from build123d import *

# Parameters (mm, degrees)
BOSS_EXTRUDE1_DEPTH = 16
SKETCH2_W           = 9
SKETCH2_H           = 16
BOSS_EXTRUDE2_DEPTH = 1
BOSS_EXTRUDE2_TAPER = 45
SKETCH3_R           = 2.6
CUT_EXTRUDE1_DEPTH  = 6
SKETCH4_R           = 1.44
BOSS_EXTRUDE3_DEPTH = 6


with BuildPart() as part:
    # Sketch1 → Boss-Extrude1 (new body)
    with BuildSketch(Plane(origin=(0, 0, 0), x_dir=(1, 0, 0), z_dir=(0, 1, 0))):
        Polygon((-6.542273602, -4.737945966), (13.457726398, -4.737945966), (9.36611498, -0.737945966), (-2.80088502, -0.737945966), align=None)
    extrude(amount=-BOSS_EXTRUDE1_DEPTH)

    # Sketch2 → Boss-Extrude2 (add)
    with BuildSketch(Plane.XY.offset(4.737945966)):
        with Locations((3.457726398, -8)):
            Rectangle(SKETCH2_W, SKETCH2_H)
    extrude(amount=BOSS_EXTRUDE2_DEPTH, taper=BOSS_EXTRUDE2_TAPER)

    # Sketch3 → Cut-Extrude1 (cut, through all)
    with BuildSketch(Plane.XY.offset(5.737945966)):
        with Locations((3.457726398, -5)):
            Circle(SKETCH3_R)
    extrude(amount=-CUT_EXTRUDE1_DEPTH, mode=Mode.SUBTRACT)

    # Sketch4 → Boss-Extrude3 (add)
    with BuildSketch(Plane.XZ.offset(16)):
        with BuildLine():
            Line((13.457726398, 4.737945966), (13.457726398, -6.650054034))
            ThreePointArc((13.457726398, -6.650054034), (10.961456039, -10.319414663), (6.631765726, -9.345066204))
            Line((6.631765726, -9.345066204), (-6.542273602, 4.737945966))
            Line((-6.542273602, 4.737945966), (13.457726398, 4.737945966))
        make_face()
        with Locations((9.512726398, -6.650054034)):
            Circle(SKETCH4_R, mode=Mode.SUBTRACT)
    extrude(amount=-BOSS_EXTRUDE3_DEPTH)


solid = part.part
CAD build for the part. Positions are in the model's coordinates, mm. A direction names the side the tool comes from. Give positions to 0.01 mm unless a question says otherwise; leave off trailing zeros. Write each loop counter-clockwise with the first axis right and the second up, starting at its lowest first coordinate (ties: lowest second). Pieces come first, ordered by that corner, then holes. Notation, with made-up numbers: (77, -24) -> (125, -24) arc R32 ccw to (125, 11) -> close; hole circle Ø6 at (-19, -8.75). An arc over 180 degrees is marked (long way). Return JSON: item names as keys, results as strings.
Item 1: Band-saw the part on A-A (y = -5). List the corners of the cut face in (x, z), then the cut area to 3 significant figures.
Answer below:
{"outline": "(-6.54, 4.74) -> (-2.8, 0.74) -> (0.86, 0.74) -> (0.86, 5.74) -> (-0.04, 5.74) -> (-1.04, 4.74) -> close; (6.06, 0.74) -> (9.37, 0.74) -> (13.46, 4.74) -> (7.96, 4.74) -> (6.96, 5.74) -> (6.06, 5.74) -> close", "area": "46.3 mm2"}
Item 2: Drill centre lines: probe 1 along Y at (x, z) = (4.5, -6.5); probe 2 along Z at (x, y) = (5, -8.25); probe 3 along Z at (x, y) = (-1.5, -7). Where is each one in solid material? Low to high.
Answer below:
{"probe 1": "y = -16 to -10", "probe 2": "z = 0.74 to 5.74", "probe 3": "z = 0.74 to 4.74"}
Item 3: Tool access for faces 1 (the flat face through (-4, -8, 4.738)), 2 (the flat face through (11.441, -4.93, 2.766)), 3 (the flat face through (3, -8, 0.738)): list every direction of +Z, -Z, +X, -X, +Y, -Y with a clear straight run to the whole face (end or side of a thin tool).
Answer below:
{"face 1": "+Z, -X, +Y, -Y", "face 2": "-Z, +X, +Y", "face 3": "-Z, +X, -X, +Y"}
Item 4: Band-saw the part on B-B (x = 1.75). List the corners of the cut face in (y, z), then the cut area to 3 significant figures.
Answer below:
{"outline": "(-16, -4.13) -> (-10, -4.13) -> (-10, 0.74) -> (-6.96, 0.74) -> (-6.96, 5.74) -> (-15, 5.74) -> (-16, 4.74) -> close; (-3.04, 0.74) -> (0, 0.74) -> (0, 4.74) -> (-1, 5.74) -> (-3.04, 5.74) -> close", "area": "88.6 mm2"}
Item 5: Drop flat-ended pins along their axis: pin 1 (6 mm diameter, centred on x = -4, y = -11.5, fed in from +Z); pin 2 (3 mm diameter, centred on x = 10.5, y = -10, fed in from +Z); pin 3 (8 mm diameter, centred on x = 2.5, z = -6, fed in from +Y); pin 4 (3 mm diameter, centred on x = 3.46, y = -5, fed in from +Z). Give the stop position or say it passes through.
Answer below:
{"pin 1": "stops at z = 4.78", "pin 2": "stops at z = 4.74", "pin 3": "stops at y = -10", "pin 4": "passes through"}
Item 6: Two-plate mould, pull along X, no slides. Class faces 4 (the cylindrical face through (10.177, -13.042, -7.928)), 5 (the flat face through (13.458, -13, -1)), 6 (the cylindrical face through (0.86, -4.89, 3.27)), 7 (the flat face through (3.52, -15.51, 5.23)): +X half, -X half, draft (parallel to the pull), parting line (faces both ways), or undercut.
Answer below:
{"face 4": "undercut", "face 5": "+X half", "face 6": "undercut", "face 7": "draft"}
Item 7: Band-saw the part on D-D (z = 1). List the corners of the cut face in (x, y).
Answer below:
{"outline": "(-3.05, -16) -> (13.46, -16) -> (13.46, -10) -> (9.63, -10) -> (9.63, 0) -> (-3.05, 0) -> close; hole circle Ø5.2 at (3.46, -5)"}
